from build123d import *

# Parameters (mm, degrees)
F0_W     = 197.0480888034
F0_H     = 6
F0_W_2   = 7.9519111966
F0_H_2   = 13.5
F0_W_3   = 1.5
F0_H_3   = 1.5
F1_DEPTH = 250
F3_DEPTH = 25
F4_R     = 2.99999


# Not quite as in the source:
# - a fillet or chamfer is up to 0.001 mm smaller than in the source, because OpenCascade refuses the exact size


with BuildPart() as f1:
    # F0 (on Top) → F1 (new body)
    with BuildSketch(Plane.XY):
        with Locations((106.4759555983, 3)):
            Rectangle(F0_W, F0_H)
        with Locations((3.9759555983, 12.75)):
            Rectangle(F0_W_2, F0_H_2)
        with Locations((3.9759555983, 3)):
            Rectangle(F0_W_2, F0_H)
        with Locations((3.9759555983, 22.5)):
            Rectangle(F0_W_2, F0_H)
        Polygon((7.9519111966, 25.5), (7.9519111966, 19.5), (30.5, 19.5), (32, 19.5), (32, 25.5), align=None)
        with Locations((31.25, 18.75)):
            Rectangle(F0_W_3, F0_H_3)
    extrude(amount=F1_DEPTH)

    # F2 (on face) → F3 (cut)
    with BuildSketch(Plane.XZ):
        Polygon((87.3010246393, 35.425593216), (108.7266178553, 14), (130.1522110713, 35.425593216), (108.7266178553, 56.851186432), align=None)
        Polygon((146.474054042, 35.425593216), (167.8996472581, 14), (189.3252404741, 35.425593216), (167.8996472581, 56.851186432), align=None)
        Polygon((149.1576427927, 95.8152501475), (167.8996472581, 77.0732456821), (186.6416517235, 95.8152501475), (167.8996472581, 114.5572546129), align=None)
        Polygon((87.3569478805, 93.1875846381), (108.7266178553, 71.8179146634), (130.09628783, 93.1875846381), (108.7266178553, 114.5572546129), align=None)
        Polygon((87.3010246393, 152.8602018807), (108.7266178553, 131.4346086647), (130.1522110713, 152.8602018807), (108.7266178553, 174.2857950967), align=None)
        Polygon((146.474054042, 152.8602018807), (167.8996472581, 131.4346086647), (189.3252404741, 152.8602018807), (167.8996472581, 174.2857950967), align=None)
        Polygon((146.474054042, 217.7387669785), (167.8996472581, 196.3131737625), (189.3252404741, 217.7387669785), (167.8996472581, 239.1643601945), align=None)
        Polygon((87.3010246393, 217.7387669785), (108.7266178553, 196.3131737625), (130.1522110713, 217.7387669785), (108.7266178553, 239.1643601945), align=None)
    extrude(amount=-F3_DEPTH, mode=Mode.SUBTRACT)

    # F4 (radius 3 in the source; OpenCascade refuses exactly that, so slightly less here)
    f4_edges = [f1.edges().sort_by_distance(p)[0] for p in [
        (205, 0, 125),
        (205, 6, 125),
        (205, 3, 0),
        (205, 3, 250),
    ]]
    fillet(f4_edges, radius=F4_R)


solid = f1.part
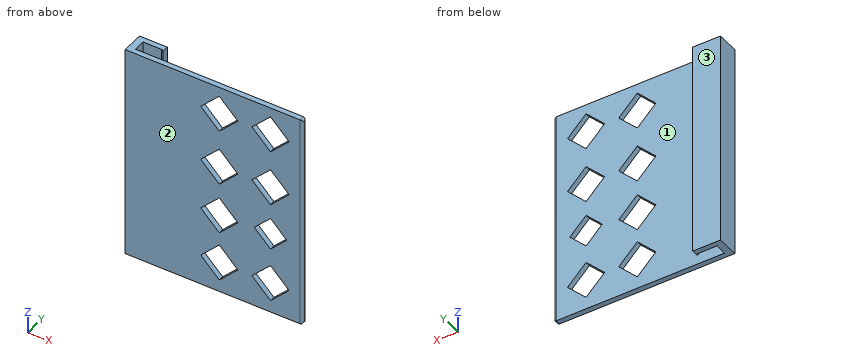
Work out the finished part from the listing and answer in its coordinate system (mm). Face numbers are marked on the shaded views. Round coordinates to 2 decimals unless told otherwise and drop trailing zeros. Order: outer loops, then holes, each group sorted by start corner. A loop starts at its lowest first (then second) coordinate and runs counter-clockwise, first axis right, second up. Notation, with made-up numbers: M 77.25,71 L 119.25,71 A17 cw 119.25,100 Z; hole C -15.5,57.5 d5. An arc over 180 degrees is marked long. Put each result on its own line as item: value. Start each with the question number.
Q1. For a pull along Y with two mould halves and no side action, classify the marked faces 1, 2 and 3 as pulls with the +Y half, pulls with the -Y half, needs draft (parallel to the pull), parting line crosses it, or undercut.
Q2. Straight lines are drawn through the part: L1, parallel to X at y = 18.25, z = 31.5; L2, parallel to Y at x = 18, z = 114; L3, parallel to X at y = 8.75, z = 206. For each, find the intervals that lie inside material, in ascending order. Write a range as [from, to].
Q3. Section D-D, the plane y = 15.25 is taken. Write down the section's boundary in (x, z), and give its area (3 significant figures).
Q4. Section A-A, the plane x = 16.5 is taken. Write down the section's boundary in (y, z).
Q5. Section B-B, the plane z = 207 is taken. Give the number of separate pieces and of enclosed holes in the cut face, and give its area (3 significant figures).
Q6. Flat-ended cylindrical pins translate along their axes: pin 1 (3 mm diameter, centred on x = 153.5, z = 27.5, fed in from +Y); pin 2 (0.8 mm diameter, centred on x = 31, z = 85, fed in from -Y); pin 3 (11 mm diameter, centred on y = 16, z = 138, fed in from +X); pin 4 (3 mm diameter, centred on y = 8, z = 171, fed in from +X). Find the tip coordinate at first contact, or state that the pin passes through.
Q7. Section C-C, the plane x = 95 is taken. Write down the section's boundary in (y, z).
Findings below:
1. face 1: undercut
1. face 2: pulls with the -Y half
1. face 3: pulls with the +Y half
2. L1: x = [0, 7.95], [30.5, 32]
2. L2: y = [0, 6], [19.5, 25.5]
2. L3: x = [0, 7.95]
3. outline: M 0,0 L 7.95,0 L 7.95,250 L 0,250 Z
3. area: 1,990 mm^2
4. outline: M 0,0 L 6,0 L 6,250 L 0,250 Z; M 19.5,0 L 25.5,0 L 25.5,250 L 19.5,250 Z
5. separate pieces: 3
5. enclosed holes: 0
5. area: 1,270 mm^2
6. pin 1: stops at y = 6
6. pin 2: stops at y = 0
6. pin 3: stops at x = 32
6. pin 4: stops at x = 7.95
7. outline: M 0,0 L 6,0 L 6,27.73 L 0,27.73 Z; M 0,43.12 L 6,43.12 L 6,85.54 L 0,85.54 Z; M 0,100.83 L 6,100.83 L 6,145.16 L 0,145.16 Z; M 0,160.56 L 6,160.56 L 6,210.04 L 0,210.04 Z; M 0,225.44 L 6,225.44 L 6,250 L 0,250 Z
